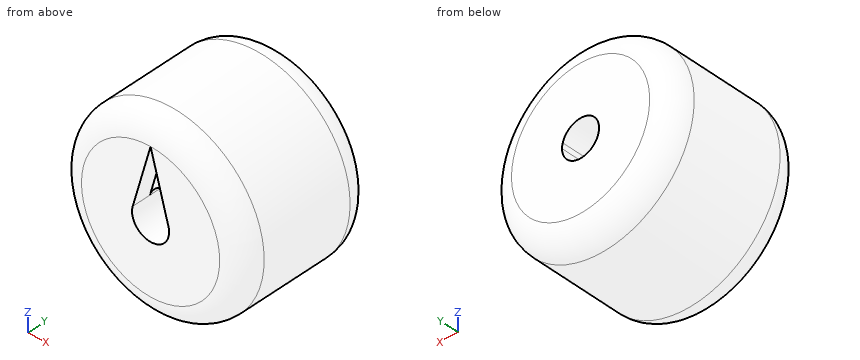
from build123d import *

# Parameters (mm, degrees)
F0_R     = 10
F0_R_2   = 9
F1_DEPTH = 15
F2_R     = 2.5
F4_DEPTH = 50
F5_DEPTH = 2


with BuildPart() as f1:
    # F0 (on Front) → F1 (new body)
    with BuildSketch(Plane.XZ):
        Circle(F0_R)
        Circle(F0_R_2, mode=Mode.SUBTRACT)
        Circle(F0_R_2)
    extrude(amount=F1_DEPTH)

    # F2
    f2_edges = [f1.edges().sort_by_distance(p)[0] for p in [
        (-10, -15, 0),
        (-10, 0, 0),
    ]]
    fillet(f2_edges, radius=F2_R)

    # F3 (on face) → F4 (cut)
    with BuildSketch(Plane.XZ.offset(15)):
        with BuildLine():
            ThreePointArc((-1.936537, 0.538719), (-0.271857, -1.991604), (2.010073, 0))
            ThreePointArc((2.010073, 0), (1.991604, 0.271857), (1.936537, 0.538719))
            ThreePointArc((1.936537, 0.538719), (0, 2.010073), (-1.936537, 0.538719))
        make_face()
    extrude(amount=-F4_DEPTH, mode=Mode.SUBTRACT)

    # F3 (on face) → F5 (cut)
    with BuildSketch(Plane.XZ.offset(15)):
        with BuildLine():
            ThreePointArc((-1.936537, 0.538719), (0, 2.010073), (1.936537, 0.538719))
            Line((1.936537, 0.538719), (0, 7.5))
            Line((0, 7.5), (-1.936537, 0.538719))
        make_face()
    extrude(amount=-F5_DEPTH, mode=Mode.SUBTRACT)


solid = f1.part
Input: part model. Units: mm. Frame: model coordinates. Give positions to 0.01 mm unless a question says otherwise; leave off trailing zeros. Write each loop counter-clockwise with the first axis right and the second up, starting at its lowest first coordinate (ties: lowest second). Pieces come first, ordered by that corner, then holes. Notation, with made-up numbers: M -20,27 L 16,27 A28 ccw 16,45 Z; hole C -17,1.25 d6. An arc over 180 degrees is marked long. Write item = value, one per line. Start each with the question number.
1) Cut plane B-B on y = -1.5. Return the cut outline in (x, z).
2) Material intervals for line 1 along Z through (x, y) = (0, -5.75); line 2 along Z through (x, y) = (1, -3.25); line 3 along Z through (x, y) = (-4, -3.5), sorted ascending. Write a range as [from, to].
3) Cut plane A-A on y = -5.75. Return the cut outline in (x, z), then the cut area to 3 significant figures.
4) First-contact query: pin 1 Ø3 at (x, y) = (6.5, -4.5) entering from +Z; pin 2 Ø1 at (y, z) = (-13.5, 0) entering from +X; pin 3 Ø2 at (y, z) = (-11, 6) entering from +X. Flat tips, straight axial feed; report the tip coordinate or a pass-through.
Solved:
q1.outline = C 0,0 d19.58; hole M 1.94,0.54 A2.01 ccw long 2.01,0 A2.01 ccw Z
q2.line_1 = [-10, -2.01], [2.01, 10]
q2.line_2 = [-9.95, -1.74], [1.74, 9.95]
q2.line_3 = [-9.17, 9.17]
q3.outline = C 0,0 d20; hole M 1.94,0.54 A2.01 ccw long 2.01,0 A2.01 ccw Z
q3.area = 301 mm2
q4.pin_1 = 8.66
q4.pin_2 = 9.95
q4.pin_3 = 8.66
